Design review of the part built by this model. Coordinates are the model's own, in mm. A direction names the side the tool comes from. Give positions to 0.01 mm unless a question says otherwise; leave off trailing zeros. Loops run counter-clockwise (first coordinate to the right, second up) from the corner with the lowest first, then second, coordinate; pieces in that order, holes last. Notation, with made-up numbers: (-6.75, 72.25) -> (46.25, 72.25) arc R25 ccw to (46.25, 109.25) -> close; hole circle Ø7 at (-23, 82.25). An arc over 180 degrees is marked (long way). Use a Markdown table: item, result. Add a question column.
1. Add section B-B (y = 267). State the section outline as (x, z) points, and give its area (3 significant figures).
2. Add section C-C (x = -14.75). State the section outline as (y, z) points.
3. For faces 1 (the flat face through (-10, 317, -594)), 2 (the flat face through (10, 135, -271)), 3 (the cylindrical face through (-14.93, 15.32, -964.54)), list the 3-axis set-ups (+Z, -Z, +X, -X, +Y, -Y) from which the entire face can be reached by the end or side of a thin tool; tool diameter is ignored.
4. To check wall thickness, follow line 1 (Z direction, x = -15, y = 300.5); line 2 (X direction, y = 419.5, z = -868); line 3 (X direction, y = 231, z = -485.5). State the ranges of each line that lie inside material, in increasing order.
5. For pin 1 Ø1.5 at (x, y) = (5, 230.5) entering from +Z; pin 2 Ø6 at (y, z) = (296, -319.5) entering from +X; pin 3 Ø1.5 at (x, z) = (3, -122.5) entering from +Y; pin 4 Ø1.5 at (x, y) = (-16, 55.5) entering from -Z, all flat-tipped, find the tip position at first contact; note any pin that passes through.
6. Add section A-A (z = -485). State the section outline as (x, y) points.
Autodesk Inventor part; units mm, degrees
ref_plane "YZ Plane" through (0, 0, 0) normal (1, 0, 0) x (0, 1, 0)
ref_plane "XZ Plane" through (0, 0, 0) normal (0, 1, 0) x (-1, 0, 0)
ref_plane "XY Plane" through (0, 0, 0) normal (0, 0, 1) x (1, 0, 0)
sketch "Sketch1" plane through (0, 0, 0) normal (1, 0, 0) x (0, 1, 0)
  line L0 (0, 0) -> (500, 0)
  line L1 (500, 0) -> (500, -10)
  line L2 (500, -10) -> (0, -10)
  line L3 (0, -10) -> (0, 0)
  line L4 (0, 0) -> (10, 0)
  line L5 (10, 0) -> (10, -1000)
  line L6 (10, -1000) -> (0, -1000)
  line L7 (0, -1000) -> (0, 0)
  arc A0 (500, 0) -> (0, -1000) centre (1931.4141, -1340.707) ccw
  dimension "d0" = 500
  dimension "d1" = 10
  dimension "d2" = 10
  dimension "d3" = 1000
extrude "Extrusion1" add sketch "Sketch1" along normal blind 10 contours L0 L5 L2 L3 | L0 A0 L2 L5 | L2 L5 A0 L7 | L2 A0 L5
sketch "Sketch2" plane through (10, 0, 0) normal (1, 0, 0) x (0, 0, -1)
  point P0 (0, 0)
sketch "Sketch3" plane through (0, 0, 0) normal (-1, 0, 0) x (0, 0, 1)
  line L0 (0, 0) -> (-1000, 0)
  line L1 (0, 0) -> (-1000, 0)
  arc A0 (-1000, 0) -> (0, 500) centre (-1340.707, 1931.4141) ccw
  line L2 (0, 500) -> (0, 0)
  line L3 (0, 500) -> (0, 0)
  line L4 (0, 500) -> (-1000, 0)
extrude "Extrusion2" add sketch "Sketch3" along normal blind 10
sketch "Sketch4" plane through (10, 0, 0) normal (1, 0, 0) x (0, 0, -1)
  line L0 (0, 500) -> (0, 0)
  line L1 (0, 500) -> (0, 0)
  line L2 (0, 0) -> (1000, 0)
  line L3 (0, 0) -> (1000, 0)
sketch "Sketch5" plane through (-10, 0, 0) normal (-1, 0, 0) x (0, 0, 1)
  line L0 (0, 0) -> (-1000, 0) construction
  line L1 (-1000, 0) -> (-950, 0) construction
  line L2 (-950, 0) -> (-950, 50) construction
  line L3 (-950, 50) -> (-1000, 50) construction
  line L4 (-1000, 50) -> (-1000, 0) construction
  arc A0 (-1000, 0) -> (-950, 50) centre (-1000.9904, 50.9904) ccw
  line L5 (-1000, 0) -> (-950, 0)
  line L6 (-950, 50) -> (-950, 0)
  dimension "d8" = 50
  dimension "d9" = 50
  dimension "d10" = 51
extrude "Extrusion3" add sketch "Sketch5" along normal blind 10
sketch "Sketch6" plane through (-10, 0, 0) normal (-1, 0, 0) x (0, 0, 1)
  line L0 (-950, 0) -> (0, 0)
  line L1 (0, 500) -> (0, 0)
  line L2 (-950, 0) -> (0, 0)
  line L3 (0, 0) -> (0, 500)
  line L4 (0, 500) -> (-950, 500)
  line L5 (-950, 500) -> (-950, 0)
extrude "Extrusion4" add sketch "Sketch6" along normal blind 10
properties part number "ramps"
Taken from the geometry:
| question | item | result |
|---|---|---|
| 1 | outline | (-20, -950) -> (-10, -950) -> (-10, -466) -> (0, -466) -> (0, -303.32) -> (10, -303.32) -> (10, 0) -> (-20, 0) -> close |
| 1 | area | 17,200 mm^2 |
| 2 | outline | (0, -1000) arc R51 cw to (50, -950) -> (500, -950) -> (500, 0) -> (0, 0) -> close |
| 3 | face 1 | -Z, +X, +Y |
| 3 | face 2 | +Z, -Z, +X, +Y, -Y |
| 3 | face 3 | -Z, -X, +Y |
| 4 | line 1 | z = -950 to 0 |
| 4 | line 2 | x = -20 to -10 |
| 4 | line 3 | x = -20 to 0 |
| 5 | pin 1 | stops at z = 0 |
| 5 | pin 2 | stops at x = 0 |
| 5 | pin 3 | stops at y = 394.99 |
| 5 | pin 4 | stops at z = -950 |
| 6 | outline | (-20, 0) -> (10, 0) -> (10, 166.7) -> (0, 166.7) -> (0, 257.5) -> (-10, 257.5) -> (-10, 500) -> (-20, 500) -> close |
